Input: part model. Units: mm. Frame: model coordinates. A direction names the side the tool comes from. Round coordinates to 2 decimals unless told otherwise and drop trailing zeros. Loops run counter-clockwise (first coordinate to the right, second up) from the corner with the lowest first, then second, coordinate; pieces in that order, holes last.
1) Section B-B, the plane x = 0. Return loops of the section in (y, z) (3 decimals), and give its area (3 significant figures).
2) Section C-C, the plane x = 22.8. Return loops of the section in (y, z) (3 decimals).
3) Draft query along Y for faces 5 (the face through (-43.05, -42.26, 1.57)), 6 (the face through (34.93, 42.05, 1.61)), 7 (the face through (14.89, -39.35, 1.61)), 8 (the face through (-7.62, -58, 2)). Return one class per face: pulls with the +Y half, pulls with the -Y half, needs draft (parallel to the pull), parting line crosses it, or undercut.
4) Section D-D, the plane y = -50.8. Return loops of the section in (x, z) (3 decimals), and give its area (3 significant figures).
5) Ray query, line 1 along X through (y, z) = (16, 1.2); line 2 along X through (y, z) = (15, 2.95); line 3 along Y through (x, z) = (33, 0.45). Return the intervals inside material, ascending.
6) First-contact query: pin 1 (1 mm diameter, centred on x = -1.5, z = 1.5, fed in from +Y); pin 2 (1 mm diameter, centred on x = 0, z = 2, fed in from -Y); pin 3 (1 mm diameter, centred on y = -9, z = 1.5, fed in from +X). Flat tips, straight axial feed; report the tip coordinate or a pass-through.
7) Access query for faces 1 (the face through (7.62, 58, 2)), 2 (the face through (-42.26, 43.05, 1.57)), 3 (the face through (-8, -36.95, 2)), 4 (the face through (58, -7.62, 2)). Directions: +Z, -Z, +X, -X, +Y, -Y. A direction counts if a zero-diameter tool reaches every point of the face in a straight line with its end or side. Return the directions, or none.
8) Section A-A, the plane y = 0. Return loops of the section in (x, z) (3 decimals).
from build123d import *

# Parameters (mm, degrees)
SKETCH1_R           = 60.325
BOSS_EXTRUDE1_DEPTH = 3.175
SKETCH2_R           = 3.175
SKETCH2_W           = 15.24
SKETCH2_H           = 6.35
CUT_EXTRUDE1_DEPTH  = 3.175
CIRPATTERN1_COUNT   = 4
SKETCH3_R           = 2
SKETCH3_R_2         = 3
CUT_EXTRUDE2_DEPTH  = 3.175
SKETCH4_R           = 2.413
CUT_EXTRUDE3_DEPTH  = 3.175
SKETCH5_R           = 3.175
BOSS_EXTRUDE2_DEPTH = 3.175
SKETCH6_R           = 1.4732
CUT_EXTRUDE4_DEPTH  = 4.175


with BuildPart() as part:
    # Sketch1 → Boss-Extrude1 (new body)
    with BuildSketch(Plane.XY):
        Circle(SKETCH1_R)
    extrude(amount=BOSS_EXTRUDE1_DEPTH)

    # Sketch2 → Cut-Extrude1 (cut)
    with BuildSketch(Plane.XY.offset(3.175)):
        with Locations((0, 50.8)):
            Circle(SKETCH2_R)
        with Locations((0, 60.325)):
            Rectangle(SKETCH2_W, SKETCH2_H)
    cut_extrude1 = extrude(amount=-CUT_EXTRUDE1_DEPTH, mode=Mode.SUBTRACT)

    # CirPattern1: Cut-Extrude1 ×4 about axis
    cirpattern1_axis = Axis((0, 0, 0), (0, 0, 1))
    for i in range(1, CIRPATTERN1_COUNT):
        add(cut_extrude1.rotate(cirpattern1_axis, i * 360 / CIRPATTERN1_COUNT), mode=Mode.SUBTRACT)

    # Sketch3 → Cut-Extrude2 (cut)
    with BuildSketch(Plane.XY.offset(3.175)):
        with Locations((-38.1, 0)):
            Circle(SKETCH3_R)
        with Locations((-29.464, 21.59)):
            Circle(SKETCH3_R)
        with Locations((-29.464, -21.59)):
            Circle(SKETCH3_R)
        with Locations((22.8, 16.945239473)):
            Circle(SKETCH3_R_2)
        with Locations((22.8, -17.054760527)):
            Circle(SKETCH3_R_2)
        Polygon((-10.1, 19.05), (-10.1, -35.95), (-10.1, -36.95), (-9.1, -36.95), (9.1, -36.95), (10.1, -36.95), (10.1, -35.95), (10.1, 2.35), (10.1, 19.05), align=None)
    extrude(amount=-CUT_EXTRUDE2_DEPTH, mode=Mode.SUBTRACT)

    # Sketch4 → Cut-Extrude3 (cut)
    with BuildSketch(Plane(origin=(0, 0, 0), x_dir=(-1, 0, 0), z_dir=(0, 0, -1))):
        with Locations((5, -34.65)):
            Circle(SKETCH4_R)
        with Locations((-5, -34.65)):
            Circle(SKETCH4_R)
        with Locations((-5, 13.35)):
            Circle(SKETCH4_R)
        with Locations((5, 13.35)):
            Circle(SKETCH4_R)
    extrude(amount=-CUT_EXTRUDE3_DEPTH, mode=Mode.SUBTRACT)

    # Sketch5 → Boss-Extrude2 (add)
    with BuildSketch(Plane(origin=(0, 0, 0), x_dir=(-1, 0, 0), z_dir=(0, 0, -1))):
        with Locations((-50.8, 0)):
            Circle(SKETCH5_R)
        with Locations((50.8, 0)):
            Circle(SKETCH5_R)
    extrude(amount=-BOSS_EXTRUDE2_DEPTH)

    # Sketch6 → Cut-Extrude4 (cut, through all)
    with BuildSketch(Plane.XY.offset(3.175)):
        with Locations((15.084311186, 40.81189221)):
            Circle(SKETCH6_R)
        with Locations((34.134311186, 40.81189221)):
            Circle(SKETCH6_R)
        with Locations((34.134311186, -40.81189221)):
            Circle(SKETCH6_R)
        with Locations((15.084311186, -40.81189221)):
            Circle(SKETCH6_R)
        with Locations((-15.084311186, -40.81189221)):
            Circle(SKETCH6_R)
        with Locations((-34.134311186, -40.81189221)):
            Circle(SKETCH6_R)
        with Locations((-34.134311186, 40.81189221)):
            Circle(SKETCH6_R)
        with Locations((-15.084311186, 40.81189221)):
            Circle(SKETCH6_R)
    extrude(amount=-CUT_EXTRUDE4_DEPTH, mode=Mode.SUBTRACT)


solid = part.part
Final values:
1. outline: (-57.15, 0) - (-53.975, 0) - (-53.975, 3.175) - (-57.15, 3.175) - close; (-47.625, 0) - (-36.95, 0) - (-36.95, 3.175) - (-47.625, 3.175) - close; (19.05, 0) - (47.625, 0) - (47.625, 3.175) - (19.05, 3.175) - close; (53.975, 0) - (57.15, 0) - (57.15, 3.175) - (53.975, 3.175) - close
1. area: 145 mm2
2. outline: (-55.85, 0) - (-20.055, 0) - (-20.055, 3.175) - (-55.85, 3.175) - close; (-14.055, 0) - (13.945, 0) - (13.945, 3.175) - (-14.055, 3.175) - close; (19.945, 0) - (55.85, 0) - (55.85, 3.175) - (19.945, 3.175) - close
3. face 5: pulls with the -Y half
3. face 6: undercut
3. face 7: undercut
3. face 8: needs draft
4. outline: (-32.534, 0) - (-3.175, 0) - (-3.175, 3.175) - (-32.534, 3.175) - close; (3.175, 0) - (32.534, 0) - (32.534, 3.175) - (3.175, 3.175) - close
4. area: 186 mm2
5. line 1: x = -58.16 to -10.1, 10.1 to 19.95, 25.65 to 58.16
5. line 2: x = -58.43 to -10.1, 10.1 to 20.52, 25.08 to 58.43
5. line 3: y = -50.5 to -41.75, -39.87 to 39.87, 41.75 to 50.5
6. pin 1: stops at y = 57.15
6. pin 2: stops at y = -57.15
6. pin 3: stops at x = 59.72
7. face 1: +Z, -Z, +Y
7. face 2: +Z, -Z, -X, +Y
7. face 3: +Z, -Z
7. face 4: +Z, -Z, +X
8. outline: (-57.15, 0) - (-40.1, 0) - (-40.1, 3.175) - (-57.15, 3.175) - close; (-36.1, 0) - (-10.1, 0) - (-10.1, 3.175) - (-36.1, 3.175) - close; (10.1, 0) - (57.15, 0) - (57.15, 3.175) - (10.1, 3.175) - close
